```python
from build123d import *

# Parameters (mm, degrees)
PAD008_DEPTH    = 7.5
SKETCH012_W     = 4.4
SKETCH012_H     = 6.5
POCKET_DEPTH    = 4.401
SKETCH013_R     = 1.75
POCKET001_DEPTH = 3.001


with BuildPart() as part:
    # Sketch011 → Pad008 (new body, symmetric)
    with BuildSketch(Plane.XZ):
        Polygon((34.6, 11.6), (39.6, 11.6), (40.4, 8.6), (40.4, 1.6), (33.8, 1.6), (33.8, 8.6), align=None)
    extrude(amount=PAD008_DEPTH, both=True)

    # Sketch012 → Pocket (cut, through all)
    with BuildSketch(Plane.YZ.offset(36)):
        with Locations((-4.85, 5.35)):
            Rectangle(SKETCH012_W, SKETCH012_H)
        with Locations((0, 5.35)):
            Rectangle(SKETCH012_W, SKETCH012_H)
        with Locations((4.85, 5.35)):
            Rectangle(SKETCH012_W, SKETCH012_H)
    extrude(amount=POCKET_DEPTH, mode=Mode.SUBTRACT)

    # Sketch013 → Pocket001 (cut, through all)
    with BuildSketch(Plane.XY.offset(8.6)):
        with Locations((37.1, -4.85)):
            Circle(SKETCH013_R)
        with Locations((37.1, 4.85)):
            Circle(SKETCH013_R)
        with Locations((37.1, 0)):
            Circle(SKETCH013_R)
    extrude(amount=POCKET001_DEPTH, mode=Mode.SUBTRACT)


solid = part.part
```
The listing builds one solid part. Answer for the finished solid, in the listing's coordinates (mm). A direction names the side the tool comes from. Give positions to 0.01 mm unless a question says otherwise; leave off trailing zeros. Order: outer loops, then holes, each group sorted by start corner. A loop starts at its lowest first (then second) coordinate and runs counter-clockwise, first axis right, second up. Notation, with made-up numbers: (81, -19) -> (109, -19) arc R8 cw to (109, -5) -> close; hole circle Ø8 at (-21.5, 63.5). An arc over 180 degrees is marked (long way). One line per item, written item: value.
1) Find section B-B, the plane z = 10.25. Determine the outline of the cut face in (x, y), plus the area to 3 significant figures.
Reported:
outline: (34.24, -7.5) -> (39.96, -7.5) -> (39.96, 7.5) -> (34.24, 7.5) -> close; hole circle Ø3.5 at (37.1, -4.85); hole circle Ø3.5 at (37.1, 0); hole circle Ø3.5 at (37.1, 4.85)
area: 56.9 mm^2
2) Find the intervals of material crossed by line 1 (Y direction, x = 39.25, z = 2.75); line 2 (Y direction, x = 37.1, z = 10.8); line 3 (Z direction, x = 38, y = 6.5), in increasing order.
Reported:
line 1: y = -7.5 to -7.05, -2.65 to -2.2, 2.2 to 2.65, 7.05 to 7.5
line 2: y = -7.5 to -6.6, -3.1 to -1.75, 1.75 to 3.1, 6.6 to 7.5
line 3: z = 1.6 to 2.1, 8.6 to 11.6
3) Flat-ended cylindrical pins translate along their axes: P1, Ø4, axis at y = -4.5, z = 10, coming from the +X side; P2, Ø1.3, axis at x = 37.5, y = -4, coming from the +Z side; P3, Ø0.5, axis at x = 36, y = 0.5, coming from the +Z side. Find the tip coordinate at first contact, or state that the pin passes through.
Reported:
P1: stops at x = 40.4
P2: stops at z = 2.1
P3: stops at z = 8.6
4) Find section C-C, the plane x = 37.1. Determine the outline of the cut face in (y, z), plus the area to 3 significant figures.
Reported:
outline: (-7.5, 1.6) -> (7.5, 1.6) -> (7.5, 11.6) -> (6.6, 11.6) -> (6.6, 8.6) -> (7.05, 8.6) -> (7.05, 2.1) -> (2.65, 2.1) -> (2.65, 8.6) -> (3.1, 8.6) -> (3.1, 11.6) -> (1.75, 11.6) -> (1.75, 8.6) -> (2.2, 8.6) -> (2.2, 2.1) -> (-2.2, 2.1) -> (-2.2, 8.6) -> (-1.75, 8.6) -> (-1.75, 11.6) -> (-3.1, 11.6) -> (-3.1, 8.6) -> (-2.65, 8.6) -> (-2.65, 2.1) -> (-7.05, 2.1) -> (-7.05, 8.6) -> (-6.6, 8.6) -> (-6.6, 11.6) -> (-7.5, 11.6) -> close
area: 32.7 mm^2
5) Find section A-A, the plane y = -4.85. Determine the outline of the cut face in (x, z), plus the area to 3 significant figures.
Reported:
outline: (33.8, 1.6) -> (40.4, 1.6) -> (40.4, 2.1) -> (36, 2.1) -> (36, 8.6) -> (35.35, 8.6) -> (35.35, 11.6) -> (34.6, 11.6) -> (33.8, 8.6) -> close; (38.85, 8.6) -> (40.4, 8.6) -> (39.6, 11.6) -> (38.85, 11.6) -> close
area: 24.5 mm^2
6) Determine the mould class of faces 4 (the flat face through (37, 7.5, 7)), 5 (the flat face through (36, 5, 5)), 6 (the flat face through (40, -0.1, 10.1)) for opening direction Y: pulls with the +Y half, pulls with the -Y half, needs draft (parallel to the pull), parting line crosses it, or undercut.
Reported:
face 4: pulls with the +Y half
face 5: undercut
face 6: needs draft
7) A tool of negligible diameter and unlimited length cuts with its end or side. For faces 1 (the flat face through (37, 0, 1.6)), 2 (the flat face through (38, 2.2, 5)), 3 (the cylindrical face through (38.717, -0.67, 10.079)), from which of +Z, -Z, +X, -X, +Y, -Y can it reach the whole face along a straight path? Write none if from no direction.
Reported:
face 1: -Z, +X, -X, +Y, -Y
face 2: +X
face 3: +Z
8) Find section D-D, the plane z = 3.5. Determine the outline of the cut face in (x, y).
Reported:
outline: (33.8, -7.5) -> (40.4, -7.5) -> (40.4, -7.05) -> (36, -7.05) -> (36, -2.65) -> (40.4, -2.65) -> (40.4, -2.2) -> (36, -2.2) -> (36, 2.2) -> (40.4, 2.2) -> (40.4, 2.65) -> (36, 2.65) -> (36, 7.05) -> (40.4, 7.05) -> (40.4, 7.5) -> (33.8, 7.5) -> close
